Part model, mm, in its own coordinate system. A direction names the side the tool comes from. Round coordinates to 2 decimals unless told otherwise and drop trailing zeros. Write each loop counter-clockwise with the first axis right and the second up, starting at its lowest first coordinate (ties: lowest second). Pieces come first, ordered by that corner, then holes.
1) Saw through at B-B on y = 15. Write the cut outline in (x, z).
2) Which spindle directions (+Z, -Z, +X, -X, +Y, -Y) get a long thin tool onto all of the face, cutting with end or side? Do faces 1 (the cylindrical face through (40.477, 7.698, 11.056)), 2 (the cylindrical face through (80.504, 15.198, 11.451)), 3 (the cylindrical face through (21.494, 15.286, 3.944)). Say none if no direction does.
3) Saw through at D-D on x = 85. Write the cut outline in (y, z), and give its area (3 significant figures).
4) Saw through at C-C on z = 10.75. Write the cut outline in (x, y), and give its area (3 significant figures).
5) Flat gauge pins, fed straight in: pin 1 (10.5 mm diameter, centred on x = 15, y = 15, fed in from +Z); pin 2 (6.5 mm diameter, centred on x = 85, y = 18, fed in from -Z); pin 3 (7 mm diameter, centred on x = 53.5, y = 19.5, fed in from +Z). Where does each tip first touch, or does it go through?
6) Saw through at A-A on x = 50. Write the cut outline in (y, z), and give its area (3 significant figures).
7) Drill centre lines: L1, parallel to X at y = 17, z = 5.5; L2, parallel to X at y = 13.5, z = 11.75; L3, parallel to Y at x = 50, z = 12. Where is each one in solid material? Low to high.
```python
from build123d import *

# Parameters (mm, degrees)
SKETCH_1_W          = 100
SKETCH_1_H          = 30
SKETCH_1_R          = 4.5
SKETCH_1_R_2        = 8
EXTRUDE_1_DEPTH     = 15
SKETCH_2_R          = 12
CUT_EXTRUDE_1_DEPTH = 8
SKETCH_3_R          = 6.5
CUT_EXTRUDE_2_DEPTH = 8
CHAMFER_1_SIZE      = 5


with BuildPart() as part:
    # 草图1 → 凸台-拉伸1 (new body)
    with BuildSketch(Plane.XY):
        with Locations((50, 15)):
            Rectangle(SKETCH_1_W, SKETCH_1_H)
        with Locations((15, 15)):
            Circle(SKETCH_1_R, mode=Mode.SUBTRACT)
        with Locations((50, 15)):
            Circle(SKETCH_1_R_2, mode=Mode.SUBTRACT)
        with Locations((85, 15)):
            Circle(SKETCH_1_R, mode=Mode.SUBTRACT)
    extrude(amount=EXTRUDE_1_DEPTH)

    # 草图2 → 切除-拉伸1 (cut)
    with BuildSketch(Plane.XY.offset(15)):
        with Locations((50, 15)):
            Circle(SKETCH_2_R)
    extrude(amount=-CUT_EXTRUDE_1_DEPTH, mode=Mode.SUBTRACT)

    # 草图3 → 切除-拉伸2 (cut)
    with BuildSketch(Plane(origin=(0, 0, 0), x_dir=(-1, 0, 0), z_dir=(0, 0, -1))):
        with Locations((-85, 15)):
            Circle(SKETCH_3_R)
        with Locations((-15, 15)):
            Circle(SKETCH_3_R)
    extrude(amount=-CUT_EXTRUDE_2_DEPTH, mode=Mode.SUBTRACT)

    # 倒角1
    chamfer_1_edges = [part.edges().sort_by_distance(p)[0] for p in [
        (0, 30, 7.5),
        (100, 30, 7.5),
        (100, 0, 7.5),
        (0, 0, 7.5),
    ]]
    chamfer(chamfer_1_edges, length=CHAMFER_1_SIZE)


solid = part.part
```
Completed:
1. outline: (0, 0) - (8.5, 0) - (8.5, 8) - (10.5, 8) - (10.5, 15) - (0, 15) - close; (19.5, 8) - (21.5, 8) - (21.5, 0) - (42, 0) - (42, 7) - (38, 7) - (38, 15) - (19.5, 15) - close; (58, 0) - (78.5, 0) - (78.5, 8) - (80.5, 8) - (80.5, 15) - (62, 15) - (62, 7) - (58, 7) - close; (89.5, 8) - (91.5, 8) - (91.5, 0) - (100, 0) - (100, 15) - (89.5, 15) - close
2. face 1: +Z
2. face 2: +Z, -Z
2. face 3: -Z
3. outline: (0, 0) - (8.5, 0) - (8.5, 8) - (10.5, 8) - (10.5, 15) - (0, 15) - close; (19.5, 8) - (21.5, 8) - (21.5, 0) - (30, 0) - (30, 15) - (19.5, 15) - close
3. area: 283 mm2
4. outline: (0, 5) - (5, 0) - (95, 0) - (100, 5) - (100, 25) - (95, 30) - (5, 30) - (0, 25) - close; hole circle Ø9 at (15, 15); hole circle Ø24 at (50, 15); hole circle Ø9 at (85, 15)
4. area: 2,370 mm2
5. pin 1: stops at z = 15
5. pin 2: stops at z = 8
5. pin 3: stops at z = 7
6. outline: (0, 0) - (7, 0) - (7, 7) - (3, 7) - (3, 15) - (0, 15) - close; (23, 0) - (30, 0) - (30, 15) - (27, 15) - (27, 7) - (23, 7) - close
6. area: 146 mm2
7. L1: x = 0 to 8.82, 21.18 to 42.25, 57.75 to 78.82, 91.18 to 100
7. L2: x = 0 to 10.76, 19.24 to 38.09, 61.91 to 80.76, 89.24 to 100
7. L3: y = 0 to 3, 27 to 30
